Geometry check sheet. Reference: the model listing, model coordinates, mm. A direction names the side the tool comes from. Give positions to 0.01 mm unless a question says otherwise; leave off trailing zeros. Loops run counter-clockwise (first coordinate to the right, second up) from the corner with the lowest first, then second, coordinate; pieces in that order, holes last. Notation, with made-up numbers: (23, 28.25) - (77, 28.25) arc R16 cw to (77, 33.25) - close; hole circle Ø7 at (-34.75, -11.5). An arc over 180 degrees is marked (long way). Use a Markdown table: item, result. Add a question column.
1. Cross-section at B-B on y = 31. Enter the section's corners in (x, z) (1 decimal), and give its area (3 significant figures).
2. Cross-section at C-C on x = 8.25. Enter the section's corners in (y, z) (3 decimals), and give its area (3 significant figures).
3. Depth check by flat-ended pin: P1, Ø1, axis at y = 8.5, z = 6.5, coming from the -X side; P2, Ø4, axis at x = 18.5, z = 7.5, coming from the -Y side; P3, Ø3, axis at y = 12, z = 7, coming from the -X side; P4, Ø5, axis at x = 13.09, z = 9.52, coming from the -Y side (3 decimals). Enter the tip coordinate at first touch or a pass-through.
4. Set-up check for faces 4 (the flat face through (5.461, 5, 9)), 5 (the cylindrical face through (9.92, 26.97, 9.66)), 6 (the flat face through (1, 9.525, 9)): record each of +Z, -Z, +X, -X, +Y, -Y from which the full face is reachable in a straight line by a thin tool's end or side.
5. Material ranges on L1, parallel to X at y = 31, z = 9.5; L2, parallel to Y at x = 23.5, z = 13.75 (3 decimals); L3, parallel to X at y = 3, z = 10, recorded low to high.
6. Cross-section at A-A on z = 11.5. Enter the section's corners in (x, y) (3 decimals), and give its area (3 significant figures).
7. Cross-section at D-D on y = 3.5. Enter the section's corners in (x, z) (1 decimal).
8. Draft check along X on faces 1 (the cylindrical face through (12.75, 31.706, 7.975)), 2 (the flat face through (26.187, 17.2, 2.5)), 3 (the flat face through (12.9, 0, 2.5)). Enter one of: pulls with the +X half, pulls with the -X half, needs draft (parallel to the pull), parting line crosses it, or undercut.
from build123d import *

# Parameters (mm, degrees)
F0_W           = 26.1874
F0_H           = 34.925
F1_DEPTH       = 15.875
F3_DEPTH       = 12.954
F4_R           = 1.5875
F5_DEPTH       = 34.926
F6_R           = 1.5875
F7_DEPTH       = 9.526
F9_D           = 3.7973
F9_CSINK_D     = 7.7978
F9_CSINK_ANGLE = 82
F10_R          = 3.175
F10_R_2        = 1.5875
F11_DEPTH      = 3.175


with BuildPart() as f1:
    # F0 (on Top) → F1 (new body)
    with BuildSketch(Plane.XY):
        with Locations((13.0937, 17.4625)):
            Rectangle(F0_W, F0_H)
    extrude(amount=F1_DEPTH)

    # F2 (on face) → F3 (cut)
    with BuildSketch(Plane.XY.offset(15.875)):
        Polygon((26.1874, 25.4), (0, 25.4), (0, 9.525), (5.461, 9.525), (5.461, 0), (20.7264, 0), (20.7264, 9.525), (26.1874, 9.525), align=None)
    extrude(amount=-F3_DEPTH, mode=Mode.SUBTRACT)

    # F4 (on face) → F5 (cut, through all)
    with BuildSketch(Plane.XZ):
        with Locations((3.175, 9.525)):
            Circle(F4_R)
        with Locations((23.0124, 9.525)):
            Circle(F4_R)
    extrude(amount=-F5_DEPTH, mode=Mode.SUBTRACT)

    # F6 (on face) → F7 (cut, through all)
    with BuildSketch(Plane.XZ.offset(-25.4)):
        with Locations((13.0937, 9.525)):
            Circle(F6_R)
    extrude(amount=-F7_DEPTH, mode=Mode.SUBTRACT)

    # F9 (through all)
    with Locations(Plane.XY.offset(2.921)):
        with Locations((13.081, 20.6502), (13.081, 9.525)):
            CounterSinkHole(F9_D / 2, F9_CSINK_D / 2, counter_sink_angle=F9_CSINK_ANGLE)

    # F10 (on face) → F11 (cut)
    with BuildSketch(Plane.XZ.offset(-25.4)):
        with Locations((13.0937, 9.525)):
            Circle(F10_R)
        with Locations((13.0937, 9.525)):
            Circle(F10_R_2, mode=Mode.SUBTRACT)
    extrude(amount=-F11_DEPTH, mode=Mode.SUBTRACT)


solid = f1.part
Values found:
| question | item | result |
|---|---|---|
| 1 | outline | (0, 0) - (26.2, 0) - (26.2, 15.9) - (0, 15.9) - close; hole circle Ø3.2 at (3.2, 9.5); hole circle Ø3.2 at (13.1, 9.5); hole circle Ø3.2 at (23, 9.5) |
| 1 | area | 392 mm2 |
| 2 | outline | (0, 0) - (34.925, 0) - (34.925, 15.875) - (25.4, 15.875) - (25.4, 2.921) - (0, 2.921) - close |
| 2 | area | 225 mm2 |
| 3 | P1 | stops at x = 0 |
| 3 | P2 | stops at y = 25.4 |
| 3 | P3 | passes through |
| 3 | P4 | stops at y = 28.575 |
| 4 | face 4 | +Z, -Y |
| 4 | face 5 | -Y |
| 4 | face 6 | +Z, +X, -X |
| 5 | L1 | x = 0 to 1.59, 4.76 to 11.51, 14.68 to 21.43, 24.6 to 26.19 |
| 5 | L2 | y = 0 to 9.525, 25.4 to 34.925 |
| 5 | L3 | x = 0 to 1.66, 4.69 to 5.46, 20.73 to 21.5, 24.53 to 26.19 |
| 6 | outline | (0, 0) - (5.461, 0) - (5.461, 9.525) - (0, 9.525) - close; (0, 25.4) - (10.608, 25.4) - (10.608, 28.575) - (15.58, 28.575) - (15.58, 25.4) - (26.187, 25.4) - (26.187, 34.925) - (0, 34.925) - close; (20.726, 0) - (26.187, 0) - (26.187, 9.525) - (20.726, 9.525) - close |
| 6 | area | 338 mm2 |
| 7 | outline | (0, 0) - (26.2, 0) - (26.2, 15.9) - (20.7, 15.9) - (20.7, 2.9) - (5.5, 2.9) - (5.5, 15.9) - (0, 15.9) - close; hole circle Ø3.2 at (3.2, 9.5); hole circle Ø3.2 at (23, 9.5) |
| 8 | face 1 | undercut |
| 8 | face 2 | pulls with the +X half |
| 8 | face 3 | needs draft |
